from build123d import *

# Parameters (mm, degrees)
SKETCH1_R           = 30
BOSS_EXTRUDE1_DEPTH = 60
SKETCH2_R           = 28.4
CUT_EXTRUDE1_DEPTH  = 58
SKETCH3_R           = 1.5
CUT_EXTRUDE2_DEPTH  = 2
FILLET2_R           = 1
FILLET3_R           = 1


with BuildPart() as part:
    # Sketch1 → Boss-Extrude1 (new body)
    with BuildSketch(Plane(origin=(0, 0, 0), x_dir=(1, 0, 0), z_dir=(0, 1, 0))):
        with Locations(Location((0, 0, 0), (0, 0, 270))):
            Circle(SKETCH1_R)
    extrude(amount=BOSS_EXTRUDE1_DEPTH)

    # Sketch2 → Cut-Extrude1 (cut)
    with BuildSketch(Plane(origin=(0, 0, 0), x_dir=(-1, 0, 0), z_dir=(0, -1, 0))):
        with Locations(Location((0, 0, 0), (0, 0, 90))):
            Circle(SKETCH2_R)
    extrude(amount=-CUT_EXTRUDE1_DEPTH, mode=Mode.SUBTRACT)

    # Sketch3 → Cut-Extrude2 (cut)
    with BuildSketch(Plane(origin=(0, 60, 0), x_dir=(1, 0, 0), z_dir=(0, 1, 0))):
        with Locations(Location((0, 0, 0), (0, 0, 270))):
            Circle(SKETCH3_R)
    extrude(amount=-CUT_EXTRUDE2_DEPTH, mode=Mode.SUBTRACT)

    # Fillet2
    fillet2_edges = [part.edges().sort_by_distance(p)[0] for p in [
        (0, 58, 28.4),
    ]]
    fillet(fillet2_edges, radius=FILLET2_R)

    # Fillet3
    fillet3_edges = [part.edges().sort_by_distance(p)[0] for p in [
        (0, 60, -30),
    ]]
    fillet(fillet3_edges, radius=FILLET3_R)


solid = part.part
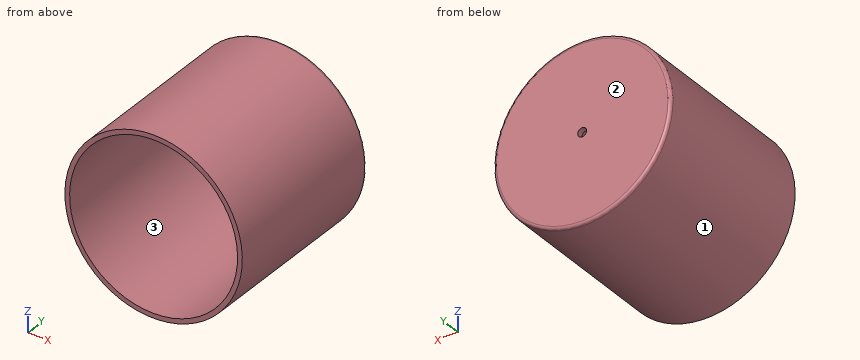
CAD build for the part. Positions are in the model's coordinates, mm. Face numbers are marked on the shaded views. Give positions to 0.01 mm unless a question says otherwise; leave off trailing zeros. Write each loop counter-clockwise with the first axis right and the second up, starting at its lowest first coordinate (ties: lowest second). Pieces come first, ordered by that corner, then holes. Notation, with made-up numbers: M 16,20 L 57,20 A16 ccw 57,41 Z; hole C 22,17.5 d2. An arc over 180 degrees is marked long. Put each result on its own line as item: value. Start each with the question number.
(1) Probe L1, parallel to Z at x = -1, y = 14.5; L2, parallel to X at y = 59, z = 0; L3, parallel to X at y = 38, z = 0. List the from-to ranges inside material, lowest first.
(2) Mould opens along X. For the marked faces 1, 2 and 3 say: +X half, -X half, draft (parallel to the pull), parting line (faces both ways), or undercut.
(3) Flat gauge pins, fed straight in: pin 1 Ø8 at (x, y) = (6, 11.5) entering from +Z; pin 2 Ø2 at (x, y) = (-1.5, 50) entering from -Z; pin 3 Ø8 at (y, z) = (46, -19.5) entering from -X. Where does each tip first touch, or does it go through?
(4) Band-saw the part on B-B, the plane x = 0. Write the cut outline in (y, z), and give its area (3 significant figures).
(5) Band-saw the part on C-C, the plane y = 35. Write the cut outline in (x, z), and give its area (3 significant figures).
(6) Band-saw the part on A-A, the plane z = 0. Write the cut outline in (x, y).
Response values:
1. L1: z = -29.98 to -28.38, 28.38 to 29.98
1. L2: x = -30 to -1.5, 1.5 to 30
1. L3: x = -30 to -28.4, 28.4 to 30
2. face 1: parting line
2. face 2: draft
2. face 3: undercut
3. pin 1: stops at z = 29.93
3. pin 2: stops at z = -30
3. pin 3: stops at x = -25.69
4. outline: M 0,-30 L 59,-30 A1 ccw 60,-29 L 60,-1.5 L 58,-1.5 L 58,-27.4 A1 cw 57,-28.4 L 0,-28.4 Z; M 0,28.4 L 57,28.4 A1 cw 58,27.4 L 58,1.5 L 60,1.5 L 60,29 A1 ccw 59,30 L 0,30 Z
4. area: 300 mm2
5. outline: C 0,0 d60; hole C 0,0 d56.8
5. area: 294 mm2
6. outline: M -30,0 L -28.4,0 L -28.4,57 A1 cw -27.4,58 L -1.5,58 L -1.5,60 L -29,60 A1 ccw -30,59 Z; M 1.5,58 L 27.4,58 A1 cw 28.4,57 L 28.4,0 L 30,0 L 30,59 A1 ccw 29,60 L 1.5,60 Z
